```python
from build123d import *

# Parameters (mm, degrees)
SKETCH1_R           = 1
BOSS_EXTRUDE1_DEPTH = 3.6


with BuildPart() as part:
    # Sketch1 → Boss-Extrude1 (new body)
    with BuildSketch(Plane.XY):
        with BuildLine():
            Line((0, 5), (12.556863352, 5))
            ThreePointArc((12.556863352, 5), (16.792661174, 7.018934049), (17.891852228, 11.580716256))
            ThreePointArc((17.891852228, 11.580716256), (19.527471102, 13.99714741), (21.883567401, 12.27575296))
            ThreePointArc((21.883567401, 12.27575296), (22.943328128, 6.983448401), (24.641136419, 1.860067939))
            ThreePointArc((24.641136419, 1.860067939), (24.141276355, -2.801754834), (20, -5))
            Line((20, -5), (0, -5))
            ThreePointArc((0, -5), (-5, 0), (0, 5))
        make_face()
        Circle(SKETCH1_R, mode=Mode.SUBTRACT)
        with Locations((20, 0)):
            Circle(SKETCH1_R, mode=Mode.SUBTRACT)
        with Locations((19.875214038, 12)):
            Circle(SKETCH1_R, mode=Mode.SUBTRACT)
    extrude(amount=BOSS_EXTRUDE1_DEPTH)


solid = part.part
```
Work out the finished part from the listing and answer in its coordinate system (mm). A direction names the side the tool comes from. Coordinates: 2 decimals unless noted, no trailing zeros. Loops run counter-clockwise (first coordinate to the right, second up) from the corner with the lowest first, then second, coordinate; pieces in that order, holes last. Notation, with made-up numbers: (44.5, 86.25) - (56.5, 86.25) arc R27 ccw to (56.5, 110.25) - close; hole circle Ø8 at (11, 68.5). An arc over 180 degrees is marked (long way). Use a Markdown table: item, result.
Item 1: The mould has two halves that part along X. Classify faces 3 (the cylindrical face through (20.8, 11.62, 1.77)), 4 (the cylindrical face through (16.75, 6.97, 1.77)), 5 (the flat face through (10, -5, 2)): +X half, -X half, draft (parallel to the pull), parting line (faces both ways), or undercut.
Evaluation:
| item | result |
|---|---|
| face 3 | undercut |
| face 4 | -X half |
| face 5 | draft |
Item 2: Find section B-B, the plane z = 3.1. Determine the outline of the cut face in (x, y).
Evaluation:
| item | result |
|---|---|
| outline | (0, -5) - (20, -5) arc R5 ccw to (24.64, 1.86) arc R44.14 cw to (21.88, 12.28) arc R2.03 ccw (long way) to (17.89, 11.58) arc R5.45 cw to (12.56, 5) - (0, 5) arc R5 ccw to start; hole circle Ø2 at (0, 0); hole circle Ø2 at (19.88, 12); hole circle Ø2 at (20, 0) |
Item 3: Given pin 1 Ø2 at (y, z) = (-1, 2) entering from -X; pin 2 Ø1.1 at (x, z) = (7, 2) entering from +Y, each flat-ended and moving along its own axis, determine where each tip first touches the part or whether it passes through.
Evaluation:
| item | result |
|---|---|
| pin 1 | stops at x = -5 |
| pin 2 | stops at y = 5 |
Item 4: Find section D-D, the plane y = 3.5. Determine the outline of the cut face in (x, z).
Evaluation:
| item | result |
|---|---|
| outline | (-3.57, 0) - (24.02, 0) - (24.02, 3.6) - (-3.57, 3.6) - close |
Item 5: Find section C-C, the plane x = -3. Determine the outline of the cut face in (y, z), and give its area (3 significant figures).
Evaluation:
| item | result |
|---|---|
| outline | (-4, 0) - (4, 0) - (4, 3.6) - (-4, 3.6) - close |
| area | 28.8 mm2 |
Item 6: Find section A-A, the plane y = 0. Determine the outline of the cut face in (x, z).
Evaluation:
| item | result |
|---|---|
| outline | (-5, 0) - (-1, 0) - (-1, 3.6) - (-5, 3.6) - close; (1, 0) - (19, 0) - (19, 3.6) - (1, 3.6) - close; (21, 0) - (25, 0) - (25, 3.6) - (21, 3.6) - close |
Item 7: For faces 1 (the cylindrical face through (0, -1, 2)), 2 (the flat face through (6, 5, 2)), determine the directions among +Z, -Z, +X, -X, +Y, -Y from which every point of the face is accessible in a straight line to the end or side of a thin tool.
Evaluation:
| item | result |
|---|---|
| face 1 | +Z, -Z |
| face 2 | +Z, -Z, -X, +Y |
Item 8: Consider probe 1 along Y at (x, z) = (20, 0.8); probe 2 along Y at (x, z) = (7.75, 0.95); probe 3 along X at (y, z) = (-0.5, 1.15). Determine where each line is inside the solid, lowest interval first. Write a range as from..to.
Evaluation:
| item | result |
|---|---|
| probe 1 | y = -5..-1, 1..11.01, 12.99..14.02 |
| probe 2 | y = -5..5 |
| probe 3 | x = -4.97..-0.87, 0.87..19.13, 20.87..24.97 |
